The listing builds one solid part. Answer for the finished solid, in the listing's coordinates (mm). A direction names the side the tool comes from. Round coordinates to 2 decimals unless told otherwise and drop trailing zeros. Write each loop counter-clockwise with the first axis right and the second up, starting at its lowest first coordinate (ties: lowest second). Pieces come first, ordered by that corner, then holes.
Item 1: Find section C-C on x = -27. Give the vertices of the cut face in (y, z), then the cut area to 3 significant figures.
Item 2: Find section B-B on z = 40.5. Give the vertices of the cut face in (x, y), then the cut area to 4 significant figures.
Item 3: A tool of negligible diameter and unlimited length cuts with its end or side. For faces 1 (the face through (-24.854, 0.676, 0.986)), 2 (the face through (0, -1, 2)), from which of +Z, -Z, +X, -X, +Y, -Y can it reach the whole face along a straight path? Write none if from no direction.
Item 4: Find section D-D on y = 15. Give the vertices of the cut face in (x, z), then the cut area to 3 significant figures.
Item 5: Each of these flat-tipped pins is pushed along its axis until it touches: pin 1 (5 mm diameter, centred on x = 27, y = -15, fed in from +Z); pin 2 (6 mm diameter, centred on y = -1, z = 16, fed in from +X); pin 3 (5 mm diameter, centred on y = 4, z = 28.5, fed in from -X). Where does it stop, or does it pass through?
Item 6: For a pull along X with two mould halves and no side action, classify faces 3 (the face through (28.038, -16.996, 0.986)), 4 (the face through (31, 0, 1)), 5 (the face through (-16.3, 19, 39)), 6 (the face through (24, 0, 2)) as +X half, -X half, draft (parallel to the pull), parting line (faces both ways), or undercut.
Item 7: Find the intervals of material crossed by probe 1 along X at (y, z) = (18.85, 40.5); probe 2 along X at (y, z) = (0, 0.75); probe 3 along Z at (x, y) = (15.5, 18.5), in increasing order.
Item 8: Find section A-A on x = -15.5. Give the vertices of the cut face in (y, z), then the cut area to 3 significant figures.
```python
from build123d import *

# Parameters (mm, degrees)
F0_W     = 62
F0_H     = 40
F0_R     = 2.25
F1_DEPTH = 2
F3_W     = 46
F3_H     = 44
F3_R     = 1.7
F3_R_2   = 12
F4_DEPTH = 2
F6_DEPTH = 1.5


with BuildPart() as f1:
    # F0 (on Top) → F1 (new body)
    with BuildSketch(Plane.XY):
        Rectangle(F0_W, F0_H)
        with Locations((-27, -15)):
            Circle(F0_R, mode=Mode.SUBTRACT)
        with Locations((27, -15)):
            Circle(F0_R, mode=Mode.SUBTRACT)
        with Locations((-27, 0)):
            Circle(F0_R, mode=Mode.SUBTRACT)
        with Locations((-27, 15)):
            Circle(F0_R, mode=Mode.SUBTRACT)
        with Locations((27, 0)):
            Circle(F0_R, mode=Mode.SUBTRACT)
        with Locations((27, 15)):
            Circle(F0_R, mode=Mode.SUBTRACT)
    extrude(amount=F1_DEPTH)

    # F3 (on offset) → F4 (join)
    with BuildSketch(Plane(origin=(0, 20, 0), x_dir=(-1, 0, 0), z_dir=(0, 1, 0))):
        with Locations((0, 24)):
            Rectangle(F3_W, F3_H)
        with Locations((-15.5, 9.5)):
            Circle(F3_R, mode=Mode.SUBTRACT)
        with Locations((15.5, 9.5)):
            Circle(F3_R, mode=Mode.SUBTRACT)
        with Locations((-15.5, 40.5)):
            Circle(F3_R, mode=Mode.SUBTRACT)
        with Locations((0, 25)):
            Circle(F3_R_2, mode=Mode.SUBTRACT)
        with Locations((15.5, 40.5)):
            Circle(F3_R, mode=Mode.SUBTRACT)
    extrude(amount=-F4_DEPTH)

    # F5 (on face) → F6 (join)
    with BuildSketch(Plane.YZ.offset(23)):
        Polygon((18, 2), (18, 46), (-20, 2), align=None)
    extrude(amount=-F6_DEPTH)

    # F7: F1 across plane


with BuildPart() as f1_1:
    add(f1.part)
    add(f1.part.mirror(Plane.YZ))


solid = f1_1.part
```
Check values:
1. outline: (-20, 0) - (-17.25, 0) - (-17.25, 2) - (-20, 2) - close; (-12.75, 0) - (-2.25, 0) - (-2.25, 2) - (-12.75, 2) - close; (2.25, 0) - (12.75, 0) - (12.75, 2) - (2.25, 2) - close; (17.25, 0) - (20, 0) - (20, 2) - (17.25, 2) - close
1. area: 53.0 mm2
2. outline: (-23, 13.25) - (-21.5, 13.25) - (-21.5, 18) - (-17.2, 18) - (-17.2, 20) - (-23, 20) - close; (-13.8, 18) - (13.8, 18) - (13.8, 20) - (-13.8, 20) - close; (17.2, 18) - (21.5, 18) - (21.5, 13.25) - (23, 13.25) - (23, 20) - (17.2, 20) - close
2. area: 92.65 mm2
3. face 1: +Z, -Z
3. face 2: +Z, -Y
4. outline: (-31, 0) - (-29.25, 0) - (-29.25, 2) - (-31, 2) - close; (-24.75, 0) - (24.75, 0) - (24.75, 2) - (23, 2) - (23, 42.53) - (21.5, 42.53) - (21.5, 2) - (-21.5, 2) - (-21.5, 42.53) - (-23, 42.53) - (-23, 2) - (-24.75, 2) - close; (29.25, 0) - (31, 0) - (31, 2) - (29.25, 2) - close
4. area: 228 mm2
5. pin 1: stops at z = 2
5. pin 2: stops at x = 23
5. pin 3: stops at x = -23
6. face 3: undercut
6. face 4: +X half
6. face 5: undercut
6. face 6: draft
7. probe 1: x = -23 to -17.2, -13.8 to 13.8, 17.2 to 23
7. probe 2: x = -31 to -29.25, -24.75 to 24.75, 29.25 to 31
7. probe 3: z = 0 to 7.8, 11.2 to 38.8, 42.2 to 46
8. outline: (-20, 0) - (20, 0) - (20, 7.8) - (18, 7.8) - (18, 2) - (-20, 2) - close; (18, 11.2) - (20, 11.2) - (20, 38.8) - (18, 38.8) - close; (18, 42.2) - (20, 42.2) - (20, 46) - (18, 46) - close
8. area: 154 mm2
